```python
from build123d import *

# Parameters (mm, degrees)
BOSS_EXTRUDE1_DEPTH          = 50.8
CUT_EXTRUDE2_START           = -19.05
SKETCH2_3_R                  = 6.35
CUT_EXTRUDE2_DEPTH           = 3.175
SKETCH2_R                    = 6.35
CUT_EXTRUDE3_DEPTH           = 20.05
CUT_EXTRUDE3_DEPTH_BACK      = 20.05
F_5_16_CLEARANCE_HOLE1_D     = 8.4328
F_5_16_CLEARANCE_HOLE1_DEPTH = 19.05
F_5_16_CLEARANCE_HOLE1_TIP   = 2.533468714
CUT_EXTRUDE12_DEPTH          = 20.05
CUT_EXTRUDE12_DEPTH_BACK     = 20.05


with BuildPart() as part:
    # Sketch1 → Boss-Extrude1 (new body)
    with BuildSketch(Plane.XY):
        Polygon((-19.05, 0), (19.05, 0), (19.05, 50.8), (11.1125, 50.8), (11.1125, 6.35), (-11.1125, 6.35), (-11.1125, 50.8), (-19.05, 50.8), align=None)
    extrude(amount=BOSS_EXTRUDE1_DEPTH)

    # Sketch2_3 → Cut-Extrude2 (cut)
    with BuildSketch(Plane(origin=(0, 0, 0), x_dir=(0, 0, -1), z_dir=(1, 0, 0)).offset(CUT_EXTRUDE2_START)):
        with Locations((-12.7, 26.9875)):
            Circle(SKETCH2_3_R)
    cut_extrude2 = extrude(amount=CUT_EXTRUDE2_DEPTH, mode=Mode.SUBTRACT)

    # Mirror2: Cut-Extrude2 across plane
    add(cut_extrude2.mirror(Plane(origin=(0, 0, 0), x_dir=(0, 0, 1), z_dir=(1, 0, 0))), mode=Mode.SUBTRACT)

    # Sketch2 → Cut-Extrude3 (cut, two sides)
    with BuildSketch(Plane(origin=(0, 0, 0), x_dir=(0, 0, -1), z_dir=(1, 0, 0))) as cut_extrude3_sk:
        with Locations((-12.7, 26.9875)):
            Circle(SKETCH2_R)
    extrude(amount=CUT_EXTRUDE3_DEPTH, mode=Mode.SUBTRACT)
    extrude(cut_extrude3_sk.sketch, amount=-CUT_EXTRUDE3_DEPTH_BACK, mode=Mode.SUBTRACT)

    # 5_16 Clearance Hole1
    with Locations(Plane(origin=(0, 6.35, 0), x_dir=(1, 0, 0), z_dir=(0, 1, 0))):
        with Locations((0, -38.1), (0, -12.7)):
            Hole(F_5_16_CLEARANCE_HOLE1_D / 2, depth=F_5_16_CLEARANCE_HOLE1_DEPTH)
            with Locations((0, 0, -(F_5_16_CLEARANCE_HOLE1_DEPTH + F_5_16_CLEARANCE_HOLE1_TIP / 2))):  # 118° drill point
                Cone(0, F_5_16_CLEARANCE_HOLE1_D / 2, F_5_16_CLEARANCE_HOLE1_TIP, mode=Mode.SUBTRACT)

    # Sketch28 → Cut-Extrude12 (cut, two sides)
    with BuildSketch(Plane(origin=(0, 0, 0), x_dir=(0, 0, -1), z_dir=(1, 0, 0))) as cut_extrude12_sk:
        with BuildLine():
            Line((0, 50.8), (-50.8, 50.8))
            Line((-50.8, 50.8), (-50.8, 6.35))
            ThreePointArc((-50.8, 6.35), (-49.173704114, 14.144110837), (-44.566221155, 20.6375))
            Line((-44.566221155, 20.6375), (-27.687967891, 36.297468352))
            ThreePointArc((-27.687967891, 36.297468352), (-23.689687593, 38.809652893), (-19.05, 39.6875))
            Line((-19.05, 39.6875), (-12.7, 39.6875))
            ThreePointArc((-12.7, 39.6875), (-3.719743879, 35.967756121), (0, 26.9875))
            Line((0, 26.9875), (0, 50.8))
        make_face()
    extrude(amount=CUT_EXTRUDE12_DEPTH, mode=Mode.SUBTRACT)
    extrude(cut_extrude12_sk.sketch, amount=-CUT_EXTRUDE12_DEPTH_BACK, mode=Mode.SUBTRACT)


solid = part.part
```
Can you work these out from the model? Positions are in its coordinate system, mm. A direction names the side the tool comes from. Round coordinates to 2 decimals unless told otherwise and drop trailing zeros. Loops run counter-clockwise (first coordinate to the right, second up) from the corner with the lowest first, then second, coordinate; pieces in that order, holes last.
Item 1: If we mould it in two halves opening along Z, with no side actions, what happens to faces 3 (the flat face through (-15, 39.688, 16)), 4 (the flat face through (0, 3, 50.8)), 5 (the cylindrical face through (0.55, 3.13, 8.52))? For each: +Z half, -Z half, draft (parallel to the pull), parting line (faces both ways), or undercut.
Item 2: Suppose I cut it at C-C, the plane y = 18. Write out the boundary of the cut face in (x, z).
Item 3: Please list where these lines run through material, in increasing order: L1, parallel to Z at x = 0, y = 4; L2, parallel to Y at x = 14.25, z = 12.7; L3, parallel to X at y = 16, z = 26.
Item 4: Suppose I cut it at D-D, the plane x = 17. Write out the boundary of the cut face in (y, z), then the cut area to 3 significant figures.
Item 5: Suppose I cut it at A-A, the plane x = 0. Write out the boundary of the cut face in (y, z), then the cut area to 3 significant figures.
Item 6: Which directions (+Z, -Z, +X, -X, +Y, -Y) give clear straight access to the entire face, cutting with the end or side of a thin tool? Please do faces 1 (the flat face through (19.05, 15, 25)), 2 (the flat face through (0, 6.35, 25)).
Item 7: Will this pin go through, and if not, where does the flat tip stop? pin 1 Ø6 at (x, y) = (10, 32) entering from +Z.
Item 8: Suppose I cut it at B-B, the plane z = 38.1. Write out the boundary of the cut face in (x, y), then the cut area to 3 significant figures.
Reported:
1. face 3: draft
1. face 4: +Z half
1. face 5: undercut
2. outline: (-19.05, 0) - (-11.11, 0) - (-11.11, 46.93) - (-19.05, 46.93) - close; (11.11, 0) - (19.05, 0) - (19.05, 46.93) - (11.11, 46.93) - close
3. L1: z = 0 to 8.48, 16.92 to 33.88, 42.32 to 50.8
3. L2: y = 0 to 20.64, 33.34 to 39.69
3. L3: x = -19.05 to -11.11, 11.11 to 19.05
4. outline: (0, 0) - (26.99, 0) arc R12.7 ccw to (39.69, 12.7) - (39.69, 19.05) arc R12.7 ccw to (36.3, 27.69) - (20.64, 44.57) arc R19.49 ccw to (6.35, 50.8) - (0, 50.8) - close; hole circle Ø12.7 at (26.99, 12.7)
4. area: 1,510 mm2
5. outline: (0, 0) - (6.35, 0) - (6.35, 8.48) - (0, 8.48) - close; (0, 16.92) - (6.35, 16.92) - (6.35, 33.88) - (0, 33.88) - close; (0, 42.32) - (6.35, 42.32) - (6.35, 50.8) - (0, 50.8) - close
5. area: 215 mm2
6. face 1: +Z, -Z, +X, +Y, -Y
6. face 2: +Z, -Z, +Y
7. pin 1: stops at z = 35.32
8. outline: (-19.05, 0) - (-4.22, 0) - (-4.22, 6.35) - (-11.11, 6.35) - (-11.11, 26.64) - (-19.05, 26.64) - close; (4.22, 0) - (19.05, 0) - (19.05, 26.64) - (11.11, 26.64) - (11.11, 6.35) - (4.22, 6.35) - close
8. area: 510 mm2
